CAD build for the part. Positions are in the model's coordinates, mm. Face numbers are marked on the shaded views. A direction names the side the tool comes from. Give positions to 0.01 mm unless a question says otherwise; leave off trailing zeros. Order: outer loops, then holes, each group sorted by start corner. A loop starts at its lowest first (then second) coordinate and runs counter-clockwise, first axis right, second up.
Item 1: Band-saw the part on A-A on x = 0. Give the cut face in (y, z), plus the area to 3 significant figures.
Item 2: Flat gauge pins, fed straight in: P1, Ø2.5, axis at x = 18.5, y = 31, coming from the +Z side; P2, Ø10, axis at x = 30.16, y = 0, coming from the +Z side; P3, Ø1.8, axis at y = 35.72, z = 34.29, coming from the +X side. Where does each tip first touch, or does it go through?
Item 3: Band-saw the part on B-B on y = 11. Give the cut face in (x, z), plus the area to 3 significant figures.
Item 4: Two-plate mould, pull along X, no slides. Class the marked faces 3, 4 and 5: released by +X, released by -X, zero draft, split by the parting line, or undercut.
Item 5: Band-saw the part on C-C on z = 38.1. Give the cut face in (x, y).
Item 6: Band-saw the part on D-D on x = 27.5. Give the cut face in (y, z), plus the area to 3 significant figures.
Item 7: Wall check: L1, parallel to Y at x = -19, z = 69; L2, parallel to X at y = 31.75, z = 71.5 (3 decimals); L3, parallel to X at y = -3, z = 5.5. Give the ranges that are in metal, low to high.
Item 8: Which spindle directions (+Z, -Z, +X, -X, +Y, -Y) get a long thin tool onto all of the face, cutting with end or side? Do the marked faces 1 and 2. Say none if no direction does.
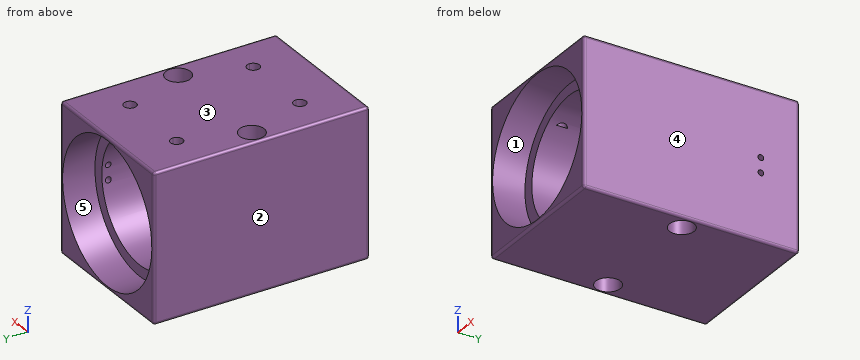
```python
from build123d import *

# Parameters (mm, degrees)
SKETCH1_W           = 76.2
SKETCH1_H           = 111.125
BOSS_EXTRUDE1_DEPTH = 76.2
SKETCH2_R           = 30.861
CUT_EXTRUDE1_DEPTH  = 127
SKETCH3_R           = 36.5125
CUT_EXTRUDE2_DEPTH  = 16.66875
CUT_EXTRUDE3_START  = -16.66875
SKETCH4_R           = 36.5125
CUT_EXTRUDE3_DEPTH  = 16.66875
SKETCH5_R           = 6.35
CUT_EXTRUDE4_DEPTH  = 102.711559846
CUT_EXTRUDE5_DEPTH  = 12.7
FILLET1_R           = 1.27
SKETCH8_R           = 1.4732
CUT_EXTRUDE6_DEPTH  = 23.622


with BuildPart() as part:
    # Sketch1 → Boss-Extrude1 (new body)
    with BuildSketch(Plane.XY):
        Rectangle(SKETCH1_W, SKETCH1_H)
    extrude(amount=BOSS_EXTRUDE1_DEPTH)

    # Sketch2 → Cut-Extrude1 (cut)
    with BuildSketch(Plane(origin=(0, 55.5625, 0), x_dir=(1, 0, 0), z_dir=(0, 1, 0))):
        with Locations(Location((0, -38.1, 0), (0, 0, 270))):
            Circle(SKETCH2_R)
    extrude(amount=-CUT_EXTRUDE1_DEPTH, mode=Mode.SUBTRACT)

    # Sketch3 → Cut-Extrude2 (cut)
    with BuildSketch(Plane(origin=(0, 55.5625, 0), x_dir=(1, 0, 0), z_dir=(0, 1, 0))):
        with Locations(Location((0, -38.1, 0), (0, 0, 270))):
            Circle(SKETCH3_R)
    extrude(amount=-CUT_EXTRUDE2_DEPTH, mode=Mode.SUBTRACT)

    # Sketch4 → Cut-Extrude3 (cut)
    with BuildSketch(Plane.XZ.offset(55.5625).offset(CUT_EXTRUDE3_START)):
        with Locations(Location((0, 38.1, 0), (0, 0, 90))):
            Circle(SKETCH4_R)
    extrude(amount=CUT_EXTRUDE3_DEPTH, mode=Mode.SUBTRACT)

    # Sketch5 → Cut-Extrude4 (cut, through all)
    with BuildSketch(Plane.XY.offset(76.2)):
        with Locations((-30.1625, 0)):
            Circle(SKETCH5_R)
        with Locations((30.1625, 0)):
            Circle(SKETCH5_R)
    extrude(amount=-CUT_EXTRUDE4_DEPTH, mode=Mode.SUBTRACT)

    # Sketch6 → Cut-Extrude5 (cut)
    with BuildSketch(Plane.XY.offset(76.2)):
        with BuildLine():
            ThreePointArc((-15.875, 31.75), (-21.29506403, 33.99506403), (-19.05, 28.575))
            Line((-19.05, 28.575), (-19.05, 31.75))
            Line((-19.05, 31.75), (-15.875, 31.75))
        make_face()
        with BuildLine():
            Line((-19.05, 31.75), (-19.05, 28.575))
            ThreePointArc((-19.05, 28.575), (-16.80493597, 29.50493597), (-15.875, 31.75))
            Line((-15.875, 31.75), (-19.05, 31.75))
        make_face()
        with BuildLine():
            ThreePointArc((15.875, 31.75), (16.80493597, 29.50493597), (19.05, 28.575))
            Line((19.05, 28.575), (19.05, 31.75))
            Line((19.05, 31.75), (15.875, 31.75))
        make_face()
        with BuildLine():
            Line((19.05, 31.75), (19.05, 28.575))
            ThreePointArc((19.05, 28.575), (21.29506403, 29.50493597), (22.225, 31.75))
            ThreePointArc((22.225, 31.75), (19.05, 34.925), (15.875, 31.75))
            Line((15.875, 31.75), (19.05, 31.75))
        make_face()
        with BuildLine():
            ThreePointArc((-19.05, -28.575), (-21.29506403, -33.99506403), (-15.875, -31.75))
            Line((-15.875, -31.75), (-19.05, -31.75))
            Line((-19.05, -31.75), (-19.05, -28.575))
        make_face()
        with BuildLine():
            Line((-19.05, -31.75), (-15.875, -31.75))
            ThreePointArc((-15.875, -31.75), (-16.80493597, -29.50493597), (-19.05, -28.575))
            Line((-19.05, -28.575), (-19.05, -31.75))
        make_face()
        with BuildLine():
            ThreePointArc((19.05, -28.575), (16.80493597, -29.50493597), (15.875, -31.75))
            Line((15.875, -31.75), (19.05, -31.75))
            Line((19.05, -31.75), (19.05, -28.575))
        make_face()
        with BuildLine():
            Line((19.05, -31.75), (15.875, -31.75))
            ThreePointArc((15.875, -31.75), (19.05, -34.925), (22.225, -31.75))
            ThreePointArc((22.225, -31.75), (21.29506403, -29.50493597), (19.05, -28.575))
            Line((19.05, -28.575), (19.05, -31.75))
        make_face()
    extrude(amount=-CUT_EXTRUDE5_DEPTH, mode=Mode.SUBTRACT)

    # Fillet1
    fillet1_edges = [part.edges().sort_by_distance(p)[0] for p in [
        (-38.1, 0, 76.2),
        (0, -55.5625, 76.2),
        (38.1, 0, 76.2),
        (0, -55.5625, 0),
        (-38.1, 0, 0),
        (0, 55.5625, 0),
        (38.1, 0, 0),
        (0, 55.5625, 76.2),
        (38.1, -55.5625, 38.1),
        (-38.1, -55.5625, 38.1),
        (-38.1, 55.5625, 38.1),
        (38.1, 55.5625, 38.1),
    ]]
    fillet(fillet1_edges, radius=FILLET1_R)

    # Sketch8 → Cut-Extrude6 (cut)
    with BuildSketch(Plane.ZY.offset(-38.1)):
        with Locations(Location((34.29, 35.71875, 0), (0, 0, 180))):
            Circle(SKETCH8_R)
        with Locations(Location((41.91, 35.71875, 0), (0, 0, 180))):
            Circle(SKETCH8_R)
    extrude(amount=CUT_EXTRUDE6_DEPTH, mode=Mode.SUBTRACT)


solid = part.part
```
The answers:
1. outline: (-55.56, 1.27) arc R1.27 ccw to (-54.29, 0) - (54.29, 0) arc R1.27 ccw to (55.56, 1.27) - (55.56, 1.59) - (38.89, 1.59) - (38.89, 7.24) - (-38.89, 7.24) - (-38.89, 1.59) - (-55.56, 1.59) - close; (-55.56, 74.61) - (-38.89, 74.61) - (-38.89, 68.96) - (38.89, 68.96) - (38.89, 74.61) - (55.56, 74.61) - (55.56, 74.93) arc R1.27 ccw to (54.29, 76.2) - (-54.29, 76.2) arc R1.27 ccw to (-55.56, 74.93) - close
1. area: 1,230 mm2
2. P1: stops at z = 63.5
2. P2: passes through
2. P3: stops at x = -30.5
3. outline: (-38.1, 1.27) arc R1.27 ccw to (-36.83, 0) - (36.83, 0) arc R1.27 ccw to (38.1, 1.27) - (38.1, 74.93) arc R1.27 ccw to (36.83, 76.2) - (-36.83, 76.2) arc R1.27 ccw to (-38.1, 74.93) - close; hole circle Ø61.72 at (0, 38.1)
3. area: 2,810 mm2
4. face 3: zero draft
4. face 4: released by +X
4. face 5: undercut
5. outline: (-38.1, -54.29) arc R1.27 ccw to (-36.83, -55.56) - (-36.51, -55.56) - (-36.51, -38.89) - (-30.86, -38.89) - (-30.86, -6.31) arc R6.35 cw to (-30.86, 6.31) - (-30.86, 38.89) - (-36.51, 38.89) - (-36.51, 55.56) - (-36.83, 55.56) arc R1.27 ccw to (-38.1, 54.29) - close; (30.86, -38.89) - (36.51, -38.89) - (36.51, -55.56) - (36.83, -55.56) arc R1.27 ccw to (38.1, -54.29) - (38.1, 54.29) arc R1.27 ccw to (36.83, 55.56) - (36.51, 55.56) - (36.51, 38.89) - (30.86, 38.89) - (30.86, 6.31) arc R6.35 cw to (30.86, -6.31) - close
6. outline: (-55.56, 1.27) arc R1.27 ccw to (-54.29, 0) - (-5.76, 0) - (-5.76, 24.09) - (-38.89, 24.09) - (-38.89, 14.08) - (-55.56, 14.08) - close; (-55.56, 62.12) - (-38.89, 62.12) - (-38.89, 52.11) - (-5.76, 52.11) - (-5.76, 76.2) - (-54.29, 76.2) arc R1.27 ccw to (-55.56, 74.93) - close; (5.76, 0) - (54.29, 0) arc R1.27 ccw to (55.56, 1.27) - (55.56, 14.08) - (38.89, 14.08) - (38.89, 24.09) - (5.76, 24.09) - close; (5.76, 52.11) - (38.89, 52.11) - (38.89, 62.12) - (55.56, 62.12) - (55.56, 74.93) arc R1.27 ccw to (54.29, 76.2) - (5.76, 76.2) - close
6. area: 4,130 mm2
7. L1: y = -38.89 to -34.92, -28.58 to 28.58, 34.92 to 38.89
7. L2: x = -38.1 to -22.225, -15.875 to 15.875, 22.225 to 38.1
7. L3: x = -38.1 to -35.76, -24.57 to 24.57, 35.76 to 38.1
8. face 1: -Y
8. face 2: +Z, -Z, -X, +Y, -Y
